Here's how the part is built. I have some questions about the finished solid (model axes, mm). Give positions to 0.01 mm unless a question says otherwise; leave off trailing zeros. Loops run counter-clockwise (first coordinate to the right, second up) from the corner with the lowest first, then second, coordinate; pieces in that order, holes last.
Q1. Will these pins go through, and if not, where does the flat tip stop? P1, Ø0.8, axis at x = 20.5, z = 0.5, coming from the +Y side; P2, Ø0.8, axis at x = -22.5, z = 0.5, coming from the -Y side; P3, Ø0.8, axis at x = 25.5, z = 1, coming from the -Y side.
Q2. I need wall thicknesses on line 1 (Y direction, x = 1, z = 1.2); line 2 (Y direction, x = -0.5, z = 1.4); line 3 (X direction, y = 21, z = 1.45). Which ranges of each line are inside material? Lowest first, please.
Q3. If we section it at B-B (y = 14.5): Give the number of separate pieces and of enclosed holes in the cut face, plus the area to 3 significant figures.
Q4. If we section it at A-A (x = 0): Please give me the cut outline in (y, z).
from build123d import *

# Parameters (mm, degrees)
F0_R     = 10
F1_DEPTH = 1.5


with BuildPart() as f1:
    # F0 (on Top) → F1 (new body)
    with BuildSketch(Plane.XY):
        with BuildLine():
            Line((-31.392589, 8.411619), (-36.705181, 9.835124))
            ThreePointArc((-36.705181, 9.835124), (-38, 0), (-36.705181, -9.835124))
            Line((-36.705181, -9.835124), (-31.392589, -8.411619))
            ThreePointArc((-31.392589, -8.411619), (-22.98097, -22.98097), (-8.411619, -31.392589))
            Line((-8.411619, -31.392589), (-9.835124, -36.705181))
            ThreePointArc((-9.835124, -36.705181), (0, -38), (9.835124, -36.705181))
            Line((9.835124, -36.705181), (8.411619, -31.392589))
            ThreePointArc((8.411619, -31.392589), (22.98097, -22.98097), (31.392589, -8.411619))
            Line((31.392589, -8.411619), (36.705181, -9.835124))
            ThreePointArc((36.705181, -9.835124), (38, 0), (36.705181, 9.835124))
            Line((36.705181, 9.835124), (31.392589, 8.411619))
            ThreePointArc((31.392589, 8.411619), (22.98097, 22.98097), (8.411619, 31.392589))
            Line((8.411619, 31.392589), (9.835124, 36.705181))
            ThreePointArc((9.835124, 36.705181), (0, 38), (-9.835124, 36.705181))
            Line((-9.835124, 36.705181), (-8.411619, 31.392589))
            ThreePointArc((-8.411619, 31.392589), (-22.98097, 22.98097), (-31.392589, 8.411619))
        make_face()
        with BuildLine():
            Line((-3, -11.101802), (-3, -30.854497))
            ThreePointArc((-3, -30.854497), (-11.863186, -28.640266), (-19.696104, -23.938745))
            Line((-19.696104, -23.938745), (-5.728839, -9.97148))
            ThreePointArc((-5.728839, -9.97148), (-4.400859, -10.624615), (-3, -11.101802))
        make_face(mode=Mode.SUBTRACT)
        with BuildLine():
            ThreePointArc((-23.938745, -19.696104), (-28.640266, -11.863186), (-30.854497, -3))
            Line((-30.854497, -3), (-11.101802, -3))
            ThreePointArc((-11.101802, -3), (-10.624615, -4.400859), (-9.97148, -5.728839))
            Line((-9.97148, -5.728839), (-23.938745, -19.696104))
        make_face(mode=Mode.SUBTRACT)
        with BuildLine():
            ThreePointArc((-20.460429, -23.288856), (-21.92031, -21.92031), (-23.288856, -20.460429))
            Line((-23.288856, -20.460429), (-9.422022, -6.593595))
            ThreePointArc((-9.422022, -6.593595), (-8.131728, -8.131728), (-6.593595, -9.422022))
            Line((-6.593595, -9.422022), (-20.460429, -23.288856))
        make_face(mode=Mode.SUBTRACT)
        with BuildLine():
            ThreePointArc((2, -30.935417), (0, -31), (-2, -30.935417))
            Line((-2, -30.935417), (-2, -11.324752))
            ThreePointArc((-2, -11.324752), (0, -11.5), (2, -11.324752))
            Line((2, -11.324752), (2, -30.935417))
        make_face(mode=Mode.SUBTRACT)
        with BuildLine():
            ThreePointArc((19.696104, -23.938745), (11.863186, -28.640266), (3, -30.854497))
            Line((3, -30.854497), (3, -11.101802))
            ThreePointArc((3, -11.101802), (4.400859, -10.624615), (5.728839, -9.97148))
            Line((5.728839, -9.97148), (19.696104, -23.938745))
        make_face(mode=Mode.SUBTRACT)
        with BuildLine():
            ThreePointArc((23.288856, -20.460429), (21.92031, -21.92031), (20.460429, -23.288856))
            Line((20.460429, -23.288856), (6.593595, -9.422022))
            ThreePointArc((6.593595, -9.422022), (8.131728, -8.131728), (9.422022, -6.593595))
            Line((9.422022, -6.593595), (23.288856, -20.460429))
        make_face(mode=Mode.SUBTRACT)
        with BuildLine():
            Line((11.101802, -3), (30.854497, -3))
            ThreePointArc((30.854497, -3), (28.640266, -11.863186), (23.938745, -19.696104))
            Line((23.938745, -19.696104), (9.97148, -5.728839))
            ThreePointArc((9.97148, -5.728839), (10.624615, -4.400859), (11.101802, -3))
        make_face(mode=Mode.SUBTRACT)
        with BuildLine():
            ThreePointArc((-30.935417, -2), (-31, 0), (-30.935417, 2))
            Line((-30.935417, 2), (-11.324752, 2))
            ThreePointArc((-11.324752, 2), (-11.5, 0), (-11.324752, -2))
            Line((-11.324752, -2), (-30.935417, -2))
        make_face(mode=Mode.SUBTRACT)
        with BuildLine():
            Line((-11.101802, 3), (-30.854497, 3))
            ThreePointArc((-30.854497, 3), (-28.640266, 11.863186), (-23.938745, 19.696104))
            Line((-23.938745, 19.696104), (-9.97148, 5.728839))
            ThreePointArc((-9.97148, 5.728839), (-10.624615, 4.400859), (-11.101802, 3))
        make_face(mode=Mode.SUBTRACT)
        with BuildLine():
            ThreePointArc((-23.288856, 20.460429), (-21.92031, 21.92031), (-20.460429, 23.288856))
            Line((-20.460429, 23.288856), (-6.593595, 9.422022))
            ThreePointArc((-6.593595, 9.422022), (-8.131728, 8.131728), (-9.422022, 6.593595))
            Line((-9.422022, 6.593595), (-23.288856, 20.460429))
        make_face(mode=Mode.SUBTRACT)
        with BuildLine():
            ThreePointArc((-19.696104, 23.938745), (-11.863186, 28.640266), (-3, 30.854497))
            Line((-3, 30.854497), (-3, 11.101802))
            ThreePointArc((-3, 11.101802), (-4.400859, 10.624615), (-5.728839, 9.97148))
            Line((-5.728839, 9.97148), (-19.696104, 23.938745))
        make_face(mode=Mode.SUBTRACT)
        Circle(F0_R, mode=Mode.SUBTRACT)
        with BuildLine():
            ThreePointArc((20.460429, 23.288856), (21.92031, 21.92031), (23.288856, 20.460429))
            Line((23.288856, 20.460429), (9.422022, 6.593595))
            ThreePointArc((9.422022, 6.593595), (8.131728, 8.131728), (6.593595, 9.422022))
            Line((6.593595, 9.422022), (20.460429, 23.288856))
        make_face(mode=Mode.SUBTRACT)
        with BuildLine():
            ThreePointArc((30.935417, 2), (31, 0), (30.935417, -2))
            Line((30.935417, -2), (11.324752, -2))
            ThreePointArc((11.324752, -2), (11.5, 0), (11.324752, 2))
            Line((11.324752, 2), (30.935417, 2))
        make_face(mode=Mode.SUBTRACT)
        with BuildLine():
            ThreePointArc((23.938745, 19.696104), (28.640266, 11.863186), (30.854497, 3))
            Line((30.854497, 3), (11.101802, 3))
            ThreePointArc((11.101802, 3), (10.624615, 4.400859), (9.97148, 5.728839))
            Line((9.97148, 5.728839), (23.938745, 19.696104))
        make_face(mode=Mode.SUBTRACT)
        with BuildLine():
            Line((2, 30.935417), (2, 11.324752))
            ThreePointArc((2, 11.324752), (0, 11.5), (-2, 11.324752))
            Line((-2, 11.324752), (-2, 30.935417))
            ThreePointArc((-2, 30.935417), (0, 31), (2, 30.935417))
        make_face(mode=Mode.SUBTRACT)
        with BuildLine():
            Line((3, 11.101802), (3, 30.854497))
            ThreePointArc((3, 30.854497), (11.863186, 28.640266), (19.696104, 23.938745))
            Line((19.696104, 23.938745), (5.728839, 9.97148))
            ThreePointArc((5.728839, 9.97148), (4.400859, 10.624615), (3, 11.101802))
        make_face(mode=Mode.SUBTRACT)
    extrude(amount=F1_DEPTH)


solid = f1.part
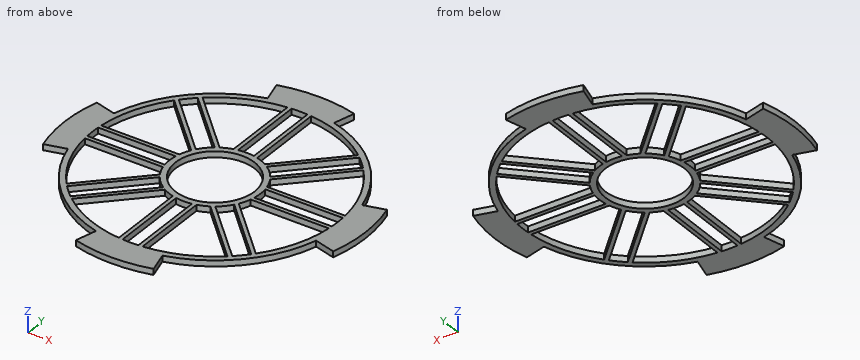
Check sheet entries:
1. P1: stops at y = 25.54
1. P2: stops at y = -23.83
1. P3: stops at y = -20.65
2. line 1: y = -37.99 to -30.98, -11.46 to -9.95, 9.95 to 11.46, 30.98 to 37.99
2. line 2: y = -38 to -31, -11.49 to -9.99, 9.99 to 11.49, 31 to 38
2. line 3: x = -24.8 to -22.8, -18.17 to -16.76, -3 to -2, 2 to 3, 16.76 to 18.17, 22.8 to 24.8
3. separate pieces: 8
3. enclosed holes: 0
3. area: 16.5 mm2
4. outline: (-38, 0) - (-31, 0) - (-31, 1.5) - (-38, 1.5) - close; (-11.5, 0) - (-10, 0) - (-10, 1.5) - (-11.5, 1.5) - close; (10, 0) - (11.5, 0) - (11.5, 1.5) - (10, 1.5) - close; (31, 0) - (38, 0) - (38, 1.5) - (31, 1.5) - close
